For this review, use the dimensioned drawing (mm, ordinates from the lowest corner) and the shaded views. Give positions to 0.01 mm unless a question says otherwise; leave off trailing zeros. Order: outer loops, then holes, each group sorted by start corner. A loop starts at its lowest first (then second) coordinate and runs counter-clockwise, first axis right, second up. Notation, with made-up numbers: (64.25, 47) -> (113.25, 47) arc R33 cw to (113.25, 84) -> close; hole circle Ø1 at (-5.5, 36). An arc over 180 degrees is marked (long way). Return JSON: item names as keys, results as strings.
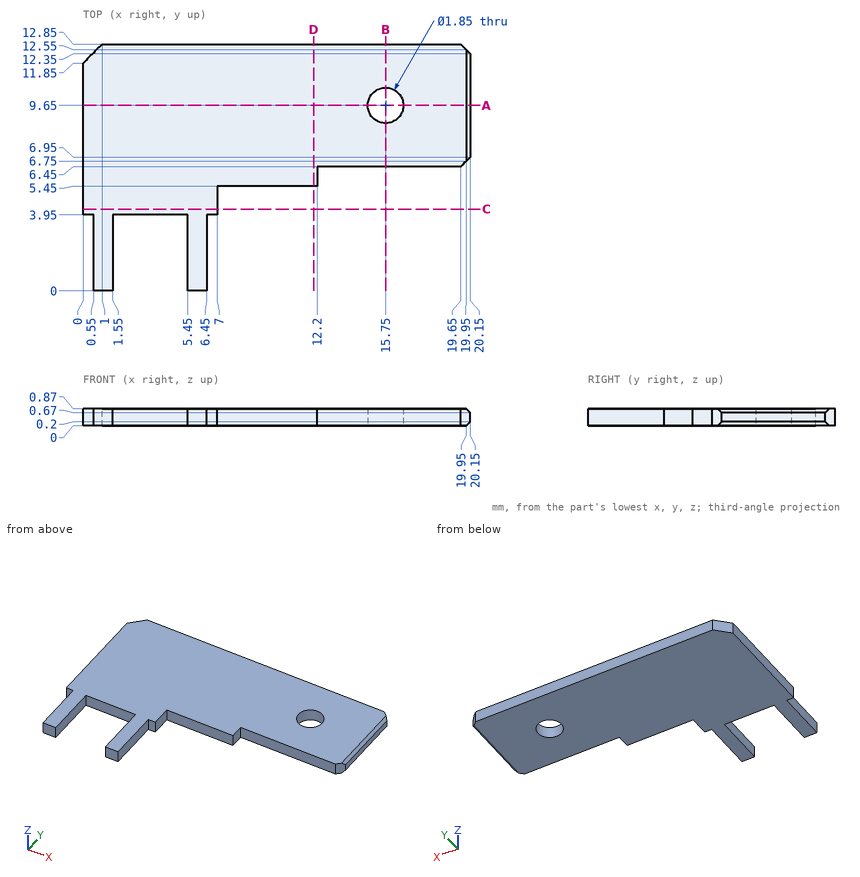
Item 1: Add section C-C (y = 4.25). Give the boundary of the cut face in (x, z), plus the area to 3 significant figures.
Result set:
{"outline": "(0, 0) -> (7, 0) -> (7, 0.87) -> (0, 0.87) -> close", "area": "6.09 mm^2"}
Item 2: Add section A-A (y = 9.65). Give the boundary of the cut face in (x, z) (3 decimals).
Result set:
{"outline": "(0, 0) -> (14.825, 0) -> (14.825, 0.87) -> (0, 0.87) -> close; (16.675, 0) -> (19.95, 0) -> (20.15, 0.2) -> (20.15, 0.67) -> (19.95, 0.87) -> (16.675, 0.87) -> close"}
Item 3: Add section B-B (x = 15.75). Give the boundary of the cut face in (y, z) (3 decimals), plus the area to 3 significant figures.
Result set:
{"outline": "(6.45, 0) -> (8.725, 0) -> (8.725, 0.87) -> (6.45, 0.87) -> close; (10.575, 0) -> (12.85, 0) -> (12.85, 0.87) -> (10.575, 0.87) -> close", "area": "3.96 mm^2"}
Item 4: Add section D-D (x = 12). Give the boundary of the cut face in (y, z).
Result set:
{"outline": "(5.45, 0) -> (12.85, 0) -> (12.85, 0.87) -> (5.45, 0.87) -> close"}
Item 5: Wall thickness on L1, parallel to X at y = 9.65, z = 0.55 (3 decimals); L2, parallel to Y at x = 15.75, z = 0.6 (3 decimals); L3, parallel to X at y = 2.25, z = 0.65: over which ranges is each line inside the solid? List them lowest first. Write a range as [from, to].
Result set:
{"L1": "x = [0, 14.825], [16.675, 20.15]", "L2": "y = [6.45, 8.725], [10.575, 12.85]", "L3": "x = [0.55, 1.55], [5.45, 6.45]"}
